Design review of the part built by this model. Coordinates are the model's own, in mm. A direction names the side the tool comes from. Coordinates: 2 decimals unless noted, no trailing zeros. Write each loop counter-clockwise with the first axis right and the second up, starting at its lowest first coordinate (ties: lowest second). Pieces come first, ordered by that corner, then holes.
Q1. For pin 1 Ø3 at (y, z) = (-7, 1.5) entering from +X; pin 2 Ø0.5 at (x, z) = (-50, 2.5) entering from +Y; pin 3 Ø5 at (x, z) = (4.5, 5) entering from -Y, all flat-tipped, find the tip position at first contact; note any pin that passes through.
Q2. Take a section at D-D, the plane x = 31.5. Write out the cut boundary in (y, z), plus the area to 3 significant figures.
Q3. The part is to be moulded in two halves that separate along Y. For faces 1 (the cylindrical face through (9.786, -49.033, 4.93)), 2 (the cylindrical face through (53.185, 21.851, 4.93)), 3 (the cylindrical face through (-9.786, 49.033, 4.93)), say which applies: released by +Y, released by -Y, zero draft, split by the parting line, or undercut.
Q4. Take a section at A-A, the plane x = 0. Write out the cut boundary in (y, z), plus the area to 3 significant figures.
Q5. For L1, parallel to Y at x = 0, z = 4; L2, parallel to X at y = -51.5, z = 5.5, list the stretches that pass through material, from the lowest coordinate up.
Q6. Take a section at C-C, the plane y = 45.5. Write out the cut boundary in (x, z), plus the area to 3 significant figures.
Q7. For faces 4 (the cylindrical face through (-41.556, -27.805, 4.93)), 5 (the cylindrical face through (-0.16, -57.5, 4.93)), 6 (the cylindrical face through (-49.046, 9.723, 4.93)), 7 (the cylindrical face through (49.046, -9.723, 4.93)), list the 3-axis set-ups (+Z, -Z, +X, -X, +Y, -Y) from which the entire face can be reached by the end or side of a thin tool; tool diameter is ignored.
from build123d import *

# Parameters (mm, degrees)
BOSS_EXTRUDE1_DEPTH     = 10
SKETCH3_R               = 16.787014752
CUT_EXTRUDE6_DEPTH      = 11
CUT_EXTRUDE6_DEPTH_BACK = 35


with BuildPart() as part:
    # Sketch2 → Boss-Extrude1 (new body)
    with BuildSketch(Plane.XY):
        with BuildLine():
            ThreePointArc((-25.846784031, 42.801212077), (-19.134171618, 46.193976626), (-11.988591043, 48.541463563))
            Line((-11.988591043, 48.541463563), (-12.205075124, 49.064102368))
            ThreePointArc((-12.205075124, 49.064102368), (-22.004297361, 53.123073119), (-26.063268112, 43.323850883))
            Line((-26.063268112, 43.323850883), (-25.846784031, 42.801212077))
        make_face()
        with BuildLine():
            ThreePointArc((-7.5, 49.434299833), (0, 50), (7.5, 49.434299833))
            Line((7.5, 49.434299833), (7.5, 50))
            ThreePointArc((7.5, 50), (0, 57.5), (-7.5, 50))
            Line((-7.5, 50), (-7.5, 49.434299833))
        make_face()
        with BuildLine():
            Line((12.205075124, 49.064102368), (11.988591043, 48.541463563))
            ThreePointArc((11.988591043, 48.541463563), (19.134171618, 46.193976626), (25.846784031, 42.801212077))
            Line((25.846784031, 42.801212077), (26.063268112, 43.323850883))
            ThreePointArc((26.063268112, 43.323850883), (22.004297361, 53.123073119), (12.205075124, 49.064102368))
        make_face()
        with BuildLine():
            Line((30.0520382, 40.658639918), (29.652027776, 40.258629494))
            ThreePointArc((29.652027776, 40.258629494), (35.355339059, 35.355339059), (40.258629494, 29.652027776))
            Line((40.258629494, 29.652027776), (40.658639918, 30.0520382))
            ThreePointArc((40.658639918, 30.0520382), (40.658639918, 40.658639918), (30.0520382, 40.658639918))
        make_face()
        with BuildLine():
            Line((43.323850883, 26.063268112), (42.801212077, 25.846784031))
            ThreePointArc((42.801212077, 25.846784031), (46.193976626, 19.134171618), (48.541463563, 11.988591043))
            Line((48.541463563, 11.988591043), (49.064102368, 12.205075124))
            ThreePointArc((49.064102368, 12.205075124), (53.123073119, 22.004297361), (43.323850883, 26.063268112))
        make_face()
        with BuildLine():
            Line((50, 7.5), (49.434299833, 7.5))
            ThreePointArc((49.434299833, 7.5), (50, 0), (49.434299833, -7.5))
            Line((49.434299833, -7.5), (50, -7.5))
            ThreePointArc((50, -7.5), (57.5, 0), (50, 7.5))
        make_face()
        with BuildLine():
            Line((49.064102368, -12.205075124), (48.541463563, -11.988591043))
            ThreePointArc((48.541463563, -11.988591043), (46.193976626, -19.134171618), (42.801212077, -25.846784031))
            Line((42.801212077, -25.846784031), (43.323850883, -26.063268112))
            ThreePointArc((43.323850883, -26.063268112), (53.123073119, -22.004297361), (49.064102368, -12.205075124))
        make_face()
        with BuildLine():
            Line((40.658639918, -30.0520382), (40.258629494, -29.652027776))
            ThreePointArc((40.258629494, -29.652027776), (35.355339059, -35.355339059), (29.652027776, -40.258629494))
            Line((29.652027776, -40.258629494), (30.0520382, -40.658639918))
            ThreePointArc((30.0520382, -40.658639918), (40.658639918, -40.658639918), (40.658639918, -30.0520382))
        make_face()
        with BuildLine():
            Line((26.063268112, -43.323850883), (25.846784031, -42.801212077))
            ThreePointArc((25.846784031, -42.801212077), (19.134171618, -46.193976626), (11.988591043, -48.541463563))
            Line((11.988591043, -48.541463563), (12.205075124, -49.064102368))
            ThreePointArc((12.205075124, -49.064102368), (22.004297361, -53.123073119), (26.063268112, -43.323850883))
        make_face()
        with BuildLine():
            Line((7.5, -50), (7.5, -49.434299833))
            ThreePointArc((7.5, -49.434299833), (0, -50), (-7.5, -49.434299833))
            Line((-7.5, -49.434299833), (-7.5, -50))
            ThreePointArc((-7.5, -50), (0, -57.5), (7.5, -50))
        make_face()
        with BuildLine():
            ThreePointArc((-11.988591043, -48.541463563), (-19.134171618, -46.193976626), (-25.846784031, -42.801212077))
            Line((-25.846784031, -42.801212077), (-26.063268112, -43.323850883))
            ThreePointArc((-26.063268112, -43.323850883), (-22.004297361, -53.123073119), (-12.205075124, -49.064102368))
            Line((-12.205075124, -49.064102368), (-11.988591043, -48.541463563))
        make_face()
        with BuildLine():
            ThreePointArc((-29.652027776, -40.258629494), (-35.355339059, -35.355339059), (-40.258629494, -29.652027776))
            Line((-40.258629494, -29.652027776), (-40.658639918, -30.0520382))
            ThreePointArc((-40.658639918, -30.0520382), (-40.658639918, -40.658639918), (-30.0520382, -40.658639918))
            Line((-30.0520382, -40.658639918), (-29.652027776, -40.258629494))
        make_face()
        with BuildLine():
            ThreePointArc((-42.801212077, -25.846784031), (-46.193976626, -19.134171618), (-48.541463563, -11.988591043))
            Line((-48.541463563, -11.988591043), (-49.064102368, -12.205075124))
            ThreePointArc((-49.064102368, -12.205075124), (-53.123073119, -22.004297361), (-43.323850883, -26.063268112))
            Line((-43.323850883, -26.063268112), (-42.801212077, -25.846784031))
        make_face()
        with BuildLine():
            ThreePointArc((-49.434299833, -7.5), (-50, 0), (-49.434299833, 7.5))
            Line((-49.434299833, 7.5), (-50, 7.5))
            ThreePointArc((-50, 7.5), (-57.5, 0), (-50, -7.5))
            Line((-50, -7.5), (-49.434299833, -7.5))
        make_face()
        with BuildLine():
            ThreePointArc((-48.541463563, 11.988591043), (-46.193976626, 19.134171618), (-42.801212077, 25.846784031))
            Line((-42.801212077, 25.846784031), (-43.323850883, 26.063268112))
            ThreePointArc((-43.323850883, 26.063268112), (-53.123073119, 22.004297361), (-49.064102368, 12.205075124))
            Line((-49.064102368, 12.205075124), (-48.541463563, 11.988591043))
        make_face()
        with BuildLine():
            Line((-40.258629494, 29.652027776), (-40.658639918, 30.0520382))
            ThreePointArc((-40.658639918, 30.0520382), (-40.658639918, 40.658639918), (-30.0520382, 40.658639918))
            Line((-30.0520382, 40.658639918), (-29.652027776, 40.258629494))
            ThreePointArc((-29.652027776, 40.258629494), (35.355339059, -35.355339059), (-40.258629494, 29.652027776))
        make_face()
    extrude(amount=BOSS_EXTRUDE1_DEPTH)

    # Sketch3 → Cut-Extrude6 (cut, two sides)
    with BuildSketch(Plane.XY) as cut_extrude6_sk:
        Circle(SKETCH3_R)
    extrude(amount=CUT_EXTRUDE6_DEPTH, mode=Mode.SUBTRACT)
    extrude(cut_extrude6_sk.sketch, amount=-CUT_EXTRUDE6_DEPTH_BACK, mode=Mode.SUBTRACT)


solid = part.part
Responses:
1. pin 1: stops at x = 55.1
1. pin 2: stops at y = 25.74
1. pin 3: stops at y = -57.23
2. outline: (-41.79, 0) - (41.79, 0) - (41.79, 10) - (-41.79, 10) - close
2. area: 836 mm2
3. face 1: released by -Y
3. face 2: undercut
3. face 3: released by +Y
4. outline: (-57.5, 0) - (-16.79, 0) - (-16.79, 10) - (-57.5, 10) - close; (16.79, 0) - (57.5, 0) - (57.5, 10) - (16.79, 10) - close
4. area: 814 mm2
5. L1: y = -57.5 to -16.79, 16.79 to 57.5
5. L2: x = -24.43 to -13.83, -7.35 to 7.35, 13.83 to 24.43
6. outline: (-26.6, 0) - (26.6, 0) - (26.6, 10) - (-26.6, 10) - close
6. area: 532 mm2
7. face 4: +Z, -Z
7. face 5: +Z, -Z, -Y
7. face 6: +Z, -Z, -X
7. face 7: +Z, -Z, +X
